```python
from build123d import *

# Parameters (mm, degrees)
SKETCH13_R           = 36
BOSS_EXTRUDE11_DEPTH = 20.0406
SKETCH14_R           = 31.75
CUT_EXTRUDE2_DEPTH   = 9.525
SKETCH16_W           = 4.2672
SKETCH16_H           = 52
BOSS_EXTRUDE12_DEPTH = 2.3876
SKETCH15_R           = 19
CUT_EXTRUDE3_DEPTH   = 56.632941278


with BuildPart() as part:
    # Sketch13 → Boss-Extrude11 (new body)
    with BuildSketch(Plane(origin=(0, 0, 0), x_dir=(0, 0, -1), z_dir=(1, 0, 0))):
        with Locations(Location((0, 0, 0), (0, 0, 180))):
            Circle(SKETCH13_R)
    extrude(amount=BOSS_EXTRUDE11_DEPTH)

    # Sketch14 → Cut-Extrude2 (cut)
    with BuildSketch(Plane.ZY):
        Circle(SKETCH14_R)
    extrude(amount=-CUT_EXTRUDE2_DEPTH, mode=Mode.SUBTRACT)

    # Sketch16 → Boss-Extrude12 (add)
    with BuildSketch(Plane(origin=(20.0406, 0, 0), x_dir=(0, 0, -1), z_dir=(1, 0, 0))):
        Rectangle(SKETCH16_W, SKETCH16_H)
    extrude(amount=BOSS_EXTRUDE12_DEPTH)

    # Sketch15 → Cut-Extrude3 (cut, through all)
    with BuildSketch(Plane.ZY):
        Circle(SKETCH15_R)
    extrude(amount=-CUT_EXTRUDE3_DEPTH, mode=Mode.SUBTRACT)


solid = part.part
```
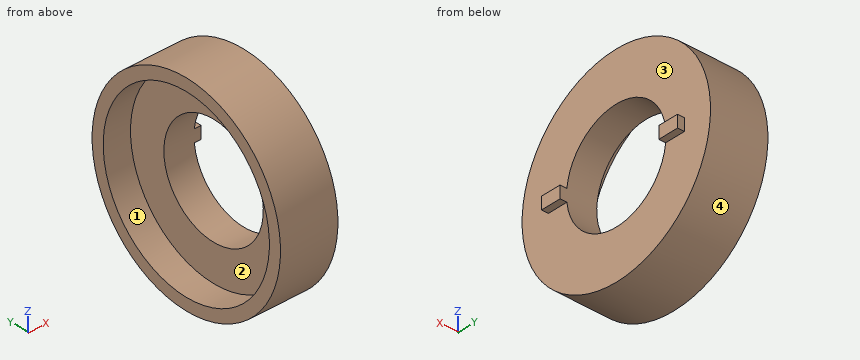
Model file for the job. Use its own axes, mm. Face numbers are marked on the shaded views. Round coordinates to 2 decimals unless told otherwise and drop trailing zeros. Write each loop counter-clockwise with the first axis right and the second up, starting at its lowest first coordinate (ties: lowest second). Pieces come first, ordered by that corner, then holes. Notation, with made-up numbers: (-33.75, 30) - (-29.75, 30) arc R12 cw to (-29.75, 34) - close; hole circle Ø10 at (24, 82.5). An arc over 180 degrees is marked (long way). Use CSV: the item, a comma, the result in double quotes. Start each with the question number.
Item 1: Drill centre lines: L1, parallel to Y at x = 7, z = 0; L2, parallel to Y at x = 6.75, z = 10.5; L3, parallel to X at y = -25, z = 0.5 (3 decimals). Where is each one in solid material? Low to high. Write a range as [from, to].
Item 2: Pin check, flat tips, straight feed: P1, Ø1.9, axis at x = 22, y = 24, coming from the +Z side; P2, Ø3, axis at x = 9.5, z = -25.5, coming from the -Y side; P3, Ø5, axis at x = 14, z = -23, coming from the +Y side. Stop position of each tip, or through.
Item 3: Band-saw the part on D-D (z = -27.5). Write the cut outline in (x, y) (3 decimals), and give its area (3 significant figures).
Item 4: Band-saw the part on A-A (y = 0). Write the cut outline in (x, z) (3 decimals).
Item 5: Two-plate mould, pull along Y, no slides. Class the marked faces 1, 2, 3 and 4: released by +Y, released by -Y, zero draft, split by the parting line, or undercut.
Item 6: Band-saw the part on B-B (z = 0). Write the cut outline in (x, y) (3 decimals), and give its area (3 significant figures).
Item 7: Band-saw the part on C-C (x = 13). Write the cut outline in (y, z), and give its area (3 significant figures).
Checked values:
1,L1,"y = [-36, -31.75], [31.75, 36]"
1,L2,"y = [-34.43, -29.96], [29.96, 34.43]"
1,L3,"x = [9.525, 22.428]"
2,P1,"stops at z = 2.13"
2,P2,"stops at y = -26.83"
2,P3,"stops at y = 29.59"
3,outline,"(0, -23.233) - (20.041, -23.233) - (20.041, 23.233) - (0, 23.233) - (0, 15.869) - (9.525, 15.869) - (9.525, -15.869) - (0, -15.869) - close"
3,area,"629 mm²"
4,outline,"(0, -36) - (20.041, -36) - (20.041, -19) - (9.525, -19) - (9.525, -31.75) - (0, -31.75) - close; (0, 31.75) - (9.525, 31.75) - (9.525, 19) - (20.041, 19) - (20.041, 36) - (0, 36) - close"
5,face 1,"undercut"
5,face 2,"undercut"
5,face 3,"zero draft"
5,face 4,"split by the parting line"
6,outline,"(0, -36) - (20.041, -36) - (20.041, -26) - (22.428, -26) - (22.428, -19) - (9.525, -19) - (9.525, -31.75) - (0, -31.75) - close; (0, 31.75) - (9.525, 31.75) - (9.525, 19) - (22.428, 19) - (22.428, 26) - (20.041, 26) - (20.041, 36) - (0, 36) - close"
6,area,"472 mm²"
7,outline,"circle Ø72 at (0, 0); hole circle Ø38 at (0, 0)"
7,area,"2,940 mm²"
